Part model, mm, in its own coordinate system. Face numbers are marked on the shaded views. A direction names the side the tool comes from. Give positions to 0.01 mm unless a question says otherwise; leave off trailing zeros. Order: outer loops, then holes, each group sorted by start corner. A loop starts at its lowest first (then second) coordinate and runs counter-clockwise, first axis right, second up. Notation, with made-up numbers: M 55,-30.5 L 105,-30.5 A13 ccw 105,-10.5 Z; hole C 75,24.25 d3. An arc over 180 degrees is marked long. Answer as a JSON object with one key per item and string values.
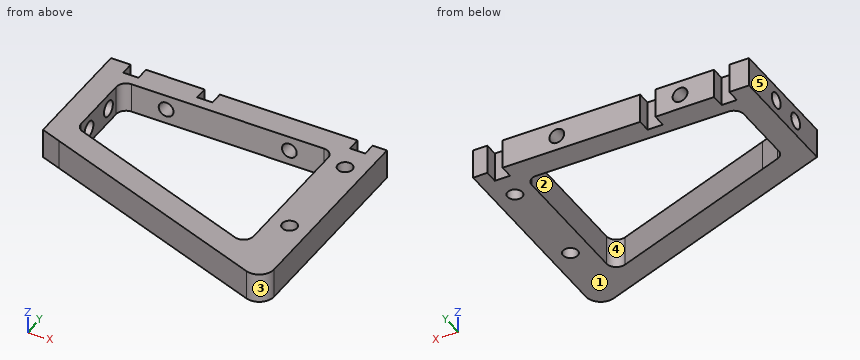
from build123d import *

# Parameters (mm, degrees)
SKETCH_1_R          = 1.5
EXTRUDE_1_DEPTH     = 6
FILLET_1_R          = 3
CUT_EXTRUDE_1_REACH = 73.29
SKETCH_2_R          = 1.5
SKETCH_3_W          = 3.1
SKETCH_3_H          = 2.7
CUT_EXTRUDE_2_DEPTH = 73.090221251
FILLET_2_R          = 2
SKETCH_4_R          = 1.6
CUT_EXTRUDE_3_DEPTH = 69.27884006


with BuildPart() as part:
    # 草图1 → 凸台-拉伸1 (new body)
    with BuildSketch(Plane.XY):
        Polygon((0, 0), (0, 45), (-56, 45), (-56, 42.266964597), (-56, 20.506230936), (-51.898147584, 19.004203562), align=None)
        with Locations((-4, 37)):
            Circle(SKETCH_1_R, mode=Mode.SUBTRACT)
        with Locations((-4, 17)):
            Circle(SKETCH_1_R, mode=Mode.SUBTRACT)
        Polygon((-51, 40), (-51, 24), (-45.845984401, 22.112688677), (-8, 8.254144103), (-8, 40), (-49, 40), align=None, mode=Mode.SUBTRACT)
    extrude(amount=EXTRUDE_1_DEPTH)

    # 圆角1
    fillet_1_edges = [part.edges().sort_by_distance(p)[0] for p in [
        (0, 0, 3),
    ]]
    fillet(fillet_1_edges, radius=FILLET_1_R)

    # 草图2 → 切除-拉伸1 (cut, up to next)
    with BuildSketch(Plane(origin=(0, 45, 0), x_dir=(1, 0, 0), z_dir=(0, 1, 0)), mode=Mode.PRIVATE) as cut_extrude_1_sk1:
        with Locations(Location((-17, -3, 0), (0, 0, 180))):
            Circle(SKETCH_2_R)
    cut_extrude_1_tool1 = extrude(cut_extrude_1_sk1.sketch, amount=-CUT_EXTRUDE_1_REACH, mode=Mode.PRIVATE) & part.part
    # 草图2 → 切除-拉伸1 (cut, up to next)
    with BuildSketch(Plane(origin=(0, 45, 0), x_dir=(1, 0, 0), z_dir=(0, 1, 0)), mode=Mode.PRIVATE) as cut_extrude_1_sk2:
        with Locations(Location((-42, -3, 0), (0, 0, 180))):
            Circle(SKETCH_2_R)
    cut_extrude_1_tool2 = extrude(cut_extrude_1_sk2.sketch, amount=-CUT_EXTRUDE_1_REACH, mode=Mode.PRIVATE) & part.part
    add(cut_extrude_1_tool1.solids().sort_by_distance((-17, 45, 3))[0], mode=Mode.SUBTRACT)
    add(cut_extrude_1_tool2.solids().sort_by_distance((-42, 45, 3))[0], mode=Mode.SUBTRACT)

    # 草图3 → 切除-拉伸2 (cut, through all)
    with BuildSketch(Plane.XY.offset(6)):
        with Locations((-50.45, 43.65)):
            Rectangle(SKETCH_3_W, SKETCH_3_H)
        with Locations((-35.45, 43.65)):
            Rectangle(SKETCH_3_W, SKETCH_3_H)
        with Locations((-4.45, 43.65)):
            Rectangle(SKETCH_3_W, SKETCH_3_H)
    extrude(amount=-CUT_EXTRUDE_2_DEPTH, mode=Mode.SUBTRACT)

    # 圆角2
    fillet_2_edges = [part.edges().sort_by_distance(p)[0] for p in [
        (-51, 40, 3),
        (-51, 24, 3),
        (-8, 8.254144103, 3),
        (-8, 40, 3),
    ]]
    fillet(fillet_2_edges, radius=FILLET_2_R)

    # 草图4 → 切除-拉伸3 (cut, through all)
    with BuildSketch(Plane(origin=(-51, 0, 0), x_dir=(0, 0, -1), z_dir=(1, 0, 0))):
        with Locations((-3, 35.198753813)):
            Circle(SKETCH_4_R)
        with Locations((-3, 28.198753813)):
            Circle(SKETCH_4_R)
    extrude(amount=-CUT_EXTRUDE_3_DEPTH, mode=Mode.SUBTRACT)


solid = part.part
1. Cut at A-A on y = 32.5. Give the cut face in (x, z).
Worked answers:
{"outline": "M -56,0 L -51,0 L -51,6 L -56,6 Z; M -8,0 L 0,0 L 0,6 L -8,6 Z"}
2. Which spindle directions (+Z, -Z, +X, -X, +Y, -Y) get a long thin tool onto all of the face, cutting with end or side? Do the marked faces 1 and 2. Say none if no direction does.
Worked answers:
{"face 1": "-Z, +X, -X, +Y, -Y", "face 2": "+Z, -Z"}
3. Cut at D-D on y = 27.5. Give the cut face in (x, z), plus the area to 3 significant figures.
Worked answers:
{"outline": "M -56,0 L -51,0 L -51,1.56 L -56,1.56 Z; M -56,4.44 L -51,4.44 L -51,6 L -56,6 Z; M -8,0 L 0,0 L 0,6 L -8,6 Z", "area": "63.6 mm^2"}
4. Cut at C-C on x = -31. Give the cut face in (y, z), plus the area to 3 significant figures.
Worked answers:
{"outline": "M 11.35,0 L 16.68,0 L 16.68,6 L 11.35,6 Z; M 40,0 L 45,0 L 45,6 L 40,6 Z", "area": "61.9 mm^2"}
5. Pin check, flat tips, straight feed: P1, Ø2.5, axis at y = 35.2, z = 3, coming from the -X side; P2, Ø1.5, axis at x = -35.5, z = 3.5, coming from the +Y side; P3, Ø3, axis at x = -21, z = 3.5, coming from the -Y side. Stop position of each tip, or through.
Worked answers:
{"P1": "stops at x = -8", "P2": "stops at y = 42.3", "P3": "stops at y = 7.14"}
6. Cut at B-B on z = 3. State how many separate pieces and enclosed holes the cut face has, plus the area to 3 significant figures.
Worked answers:
{"separate pieces": "4", "enclosed holes": "2", "area": "818 mm^2"}
7. Probe line 1 along Y through (x, z) = (-4, 4.35); line 2 along Y through (x, z) = (-53.8, 3); line 3 along Y through (x, z) = (-13, 5). List the from-to ranges inside material, lowest first.
Worked answers:
{"line 1": "y = 1.46 to 15.5, 18.5 to 35.5, 38.5 to 42.3", "line 2": "y = 19.7 to 26.6, 29.8 to 33.6, 36.8 to 45", "line 3": "y = 4.76 to 10.09, 40 to 45"}
8. Two-plate mould, pull along X, no slides. Class the marked faces 3, 4 and 5: +X half, -X half, draft (parallel to the pull), parting line (faces both ways), or undercut.
Worked answers:
{"face 3": "parting line", "face 4": "undercut", "face 5": "-X half"}
